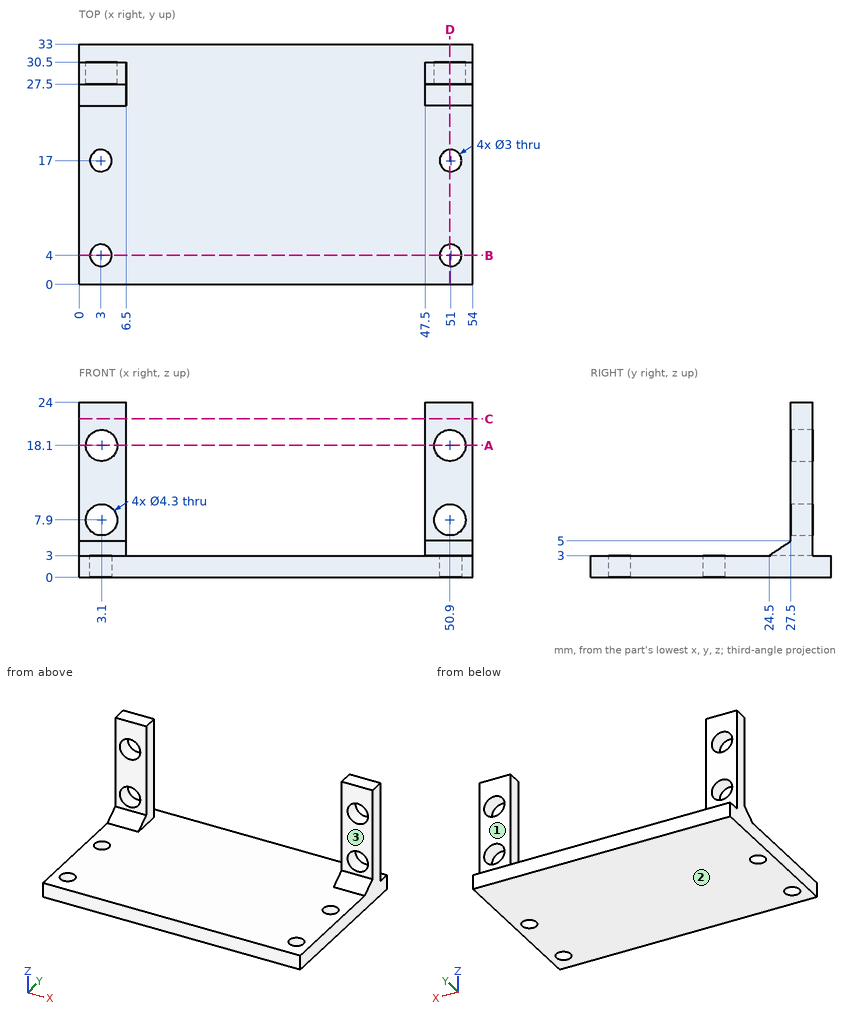
Answer from the drawing. Dimensions are ordinates in mm from the lowest x, y and z of the part. A direction names the side the tool comes from. Round coordinates to 2 decimals unless told otherwise and drop trailing zeros. Write each loop counter-clockwise with the first axis right and the second up, starting at its lowest first coordinate (ties: lowest second). Pieces come first, ordered by that corner, then holes.
1. Straight lines are drawn through the part: L1, parallel to Z at x = 3, y = 29; L2, parallel to X at y = 28.65, z = 18.1; L3, parallel to Y at x = 51, z = 1.45. For each, find the intervals that lie inside material, in ascending order.
2. Which of the six approach directions +Z, -Z, +X, -X, +Y, -Y give full straight-line access (tool end or side, diameter ignored) to the marked faces 1, 2 and 3?
3. The part is cut by section B-B, the plane y = 4. Determine the outline of the cut face in (x, z).
4. The part is cut by section D-D, the plane x = 50.9. Determine the outline of the cut face in (y, z).
5. The part is cut by section C-C, the plane z = 21.75. Determine the outline of the cut face in (x, y).
6. Given pin 1 Ø7 at (x, z) = (50.9, 7.9) entering from +Y; pin 2 Ø3 at (x, z) = (52, 10.5) entering from -Y; pin 3 Ø2.5 at (x, y) = (3, 17) entering from -Z; pin 4 Ø3.5 at (x, y) = (51, 4) entering from +Z, each flat-ended and moving along its own axis, determine where each tip first touches the part or whether it passes through.
7. The part is cut by section A-A, the plane z = 18.1. Determine the outline of the cut face in (x, y), then the cut area to 3 significant figures.
Values:
1. L1: z = 0 to 5.75, 10.05 to 15.95, 20.25 to 24
1. L2: x = 0 to 0.95, 5.25 to 6.5, 47.5 to 48.75, 53.05 to 54
1. L3: y = 0 to 2.5, 5.5 to 15.5, 18.5 to 33
2. face 1: +Z, +X, -X, +Y
2. face 2: -Z, +X, -X, +Y, -Y
2. face 3: +Z, +X, -X, -Y
3. outline: (0, 0) - (1.5, 0) - (1.5, 3) - (0, 3) - close; (4.5, 0) - (49.5, 0) - (49.5, 3) - (4.5, 3) - close; (52.5, 0) - (54, 0) - (54, 3) - (52.5, 3) - close
4. outline: (0, 0) - (2.5, 0) - (2.5, 3) - (0, 3) - close; (5.5, 0) - (15.5, 0) - (15.5, 3) - (5.5, 3) - close; (18.5, 0) - (33, 0) - (33, 3) - (30.5, 3) - (30.5, 5.75) - (27.5, 5.75) - (27.5, 5) - (24.5, 3) - (18.5, 3) - close; (27.5, 10.05) - (30.5, 10.05) - (30.5, 15.95) - (27.5, 15.95) - close; (27.5, 20.25) - (30.5, 20.25) - (30.5, 24) - (27.5, 24) - close
5. outline: (0, 27.5) - (6.5, 27.5) - (6.5, 30.5) - (0, 30.5) - close; (47.5, 27.5) - (54, 27.5) - (54, 30.5) - (47.5, 30.5) - close
6. pin 1: stops at y = 30.5
6. pin 2: stops at y = 27.5
6. pin 3: passes through
6. pin 4: stops at z = 3
7. outline: (0, 27.5) - (0.95, 27.5) - (0.95, 30.5) - (0, 30.5) - close; (5.25, 27.5) - (6.5, 27.5) - (6.5, 30.5) - (5.25, 30.5) - close; (47.5, 27.5) - (48.75, 27.5) - (48.75, 30.5) - (47.5, 30.5) - close; (53.05, 27.5) - (54, 27.5) - (54, 30.5) - (53.05, 30.5) - close
7. area: 13.2 mm2
